Source: CAD feature listing. Evaluate the final solid. Frame: model axes, mm. Give positions to 0.01 mm unless a question says otherwise; leave off trailing zeros. Order: outer loops, then holes, each group sorted by start corner. A loop starts at its lowest first (then second) coordinate and runs counter-clockwise, first axis right, second up.
from build123d import *

# Parameters (mm, degrees)
SKETCH_1_W          = 160
SKETCH_1_H          = 80
EXTRUDE_1_DEPTH     = 6
CHAMFER_1_SIZE      = 1
CHAMFER_2_SIZE      = 0.2
SKETCH_3_R          = 2
CUT_EXTRUDE_2_DEPTH = 90.643739324
CHAMFER_4_SIZE      = 0.5
FILLET_1_R          = 1


with BuildPart() as part:
    # 草图1 → 凸台-拉伸1 (new body)
    with BuildSketch(Plane(origin=(0, 0, 0), x_dir=(1, 0, 0), z_dir=(0, 1, 0))):
        Rectangle(SKETCH_1_W, SKETCH_1_H)
    extrude(amount=EXTRUDE_1_DEPTH)

    # 倒角1
    chamfer_1_edges = [part.edges().sort_by_distance(p)[0] for p in [
        (80, 6, 0),
        (0, 6, -40),
        (-80, 6, 0),
        (0, 6, 40),
    ]]
    chamfer(chamfer_1_edges, length=CHAMFER_1_SIZE)

    # 倒角2
    chamfer_2_edges = [part.edges().sort_by_distance(p)[0] for p in [
        (0, 0, -40),
        (80, 0, 0),
        (0, 0, 40),
        (-80, 0, 0),
    ]]
    chamfer(chamfer_2_edges, length=CHAMFER_2_SIZE)

    # 草图3 → 切除-拉伸2 (cut, through all)
    with BuildSketch(Plane(origin=(0, 6, 0), x_dir=(1, 0, 0), z_dir=(0, 1, 0))):
        with Locations(Location((-39, 0, 0), (0, 0, 270))):
            Circle(SKETCH_3_R)
        with Locations(Location((-4, 0, 0), (0, 0, 270))):
            Circle(SKETCH_3_R)
    extrude(amount=-CUT_EXTRUDE_2_DEPTH, mode=Mode.SUBTRACT)

    # 倒角4
    chamfer_4_edges = [part.edges().sort_by_distance(p)[0] for p in [
        (-39, 0, -2),
        (-4, 0, -2),
    ]]
    chamfer(chamfer_4_edges, length=CHAMFER_4_SIZE)

    # 圆角1
    # the kernel refuses this fillet: 1 mm, written as the material it takes off along each edge
    with BuildSketch(Plane(origin=(-80, -2.3, -40), x_dir=(1, 0, 0), z_dir=(0, 1, 0)), Plane(origin=(-80, -2.3, 40), x_dir=(0, 0, -1), z_dir=(0, 1, 0))) as fillet_1_piece_1:
        with BuildLine():
            CenterArc((FILLET_1_R, -FILLET_1_R), FILLET_1_R, 90, 90)
            Line((0, -FILLET_1_R), (0, 0))
            Line((0, 0), (FILLET_1_R, 0))
        make_face()
    extrude(amount=9.8, mode=Mode.SUBTRACT)
    with BuildSketch(Plane(origin=(80, -2.3, -40), x_dir=(-1, 0, 0), z_dir=(0, 1, 0)), Plane(origin=(80, -2.3, 40), x_dir=(0, 0, -1), z_dir=(0, 1, 0))) as fillet_1_piece_2:
        with BuildLine():
            CenterArc((FILLET_1_R, FILLET_1_R), FILLET_1_R, 180, 90)
            Line((0, FILLET_1_R), (0, 0))
            Line((0, 0), (FILLET_1_R, 0))
        make_face()
    extrude(amount=9.8, mode=Mode.SUBTRACT)


solid = part.part
1) Section query A-A on z = 0. Output: boundary loops of the cut face in (x, y), and give its area (3 significant figures).
Checks:
outline: (-80, 0.2) - (-79.8, 0) - (-41.5, 0) - (-41, 0.5) - (-41, 6) - (-79, 6) - (-80, 5) - close; (-37, 0.5) - (-36.5, 0) - (-6.5, 0) - (-6, 0.5) - (-6, 6) - (-37, 6) - close; (-2, 0.5) - (-1.5, 0) - (79.8, 0) - (80, 0.2) - (80, 5) - (79, 6) - (-2, 6) - close
area: 910 mm2
2) First-contact query: pin 1 Ø1.5 at (x, z) = (-3, -3.5) entering from -Y; pin 2 Ø3 at (x, z) = (-39, 0) entering from -Y. Flat tips, straight axial feed; report the tip coordinate or a pass-through.
Checks:
pin 1: stops at y = 0
pin 2: passes through
3) Ray query, L1, parallel to X at y = 3.7, z = 0. Return the intervals inside material, ascending.
Checks:
L1: x = -80 to -41, -37 to -6, -2 to 80
4) Pull-direction query (X, two-part tool) for faces 1 (the face through (-80, 3, 1)), 2 (the face through (-41, 3, 0)), 3 (the face through (80, 3, 1)); classes: +X half, -X half, draft (parallel to the pull), parting line (faces both ways), or undercut.
Checks:
face 1: -X half
face 2: undercut
face 3: +X half
5) Section query B-B on x = -39. Output: boundary loops of the cut face in (y, z), and give its area (3 significant figures).
Checks:
outline: (0, -39.8) - (0.2, -40) - (5, -40) - (6, -39) - (6, -2) - (0.5, -2) - (0, -2.5) - close; (0, 2.5) - (0.5, 2) - (6, 2) - (6, 39) - (5, 40) - (0.2, 40) - (0, 39.8) - close
area: 455 mm2
